from build123d import *

# Parameters (mm, degrees)
F2_SIZE2 = 1.1917535926
F2_SIZE  = 1
F3_SIZE2 = 1.1917535926
F3_SIZE  = 1
F4_SIZE  = 2
F5_SIZE2 = 1.1917535926
F5_SIZE  = 1
F6_SIZE2 = 1.1917535926
F6_SIZE  = 1


with BuildPart() as f1:
    # F0 (on Front) → F1 (revolve)
    with BuildSketch(Plane.XZ):
        Polygon((0, 30), (0, 6), (8, 6), (8, 16), (79.0824640741, 16), (91, 6), (99, 6), (99, 25), (94, 25), (92.8082464074, 24), (4, 24), (4, 30), align=None)
    revolve(axis=Axis((29.4127222821, 0, 0), (1, 0, 0)))

    # F2
    f2_edges = [f1.edges().sort_by_distance(p)[0] for p in [
        (0, 0, -6),
    ]]
    f2_side = f1.faces().sort_by_distance((0, 0, -29.151472))[0]
    chamfer(f2_edges, length=F2_SIZE, length2=F2_SIZE2, reference=f2_side)

    # F3
    f3_edges = [f1.edges().sort_by_distance(p)[0] for p in [
        (99, 0, -6),
    ]]
    f3_side = f1.faces().sort_by_distance((99, 0, -6.707107))[0]
    chamfer(f3_edges, length=F3_SIZE, length2=F3_SIZE2, reference=f3_side)

    # F4
    f4_edges = [f1.edges().sort_by_distance(p)[0] for p in [
        (99, 0, -25),
    ]]
    chamfer(f4_edges, length=F4_SIZE)

    # F5
    f5_edges = [f1.edges().sort_by_distance(p)[0] for p in [
        (0, 0, -30),
    ]]
    f5_side = f1.faces().sort_by_distance((0, 0, -7.848528))[0]
    chamfer(f5_edges, length=F5_SIZE, length2=F5_SIZE2, reference=f5_side)

    # F6
    f6_edges = [f1.edges().sort_by_distance(p)[0] for p in [
        (4, 0, -30),
    ]]
    f6_side = f1.faces().sort_by_distance((4, 0, -24.848528))[0]
    chamfer(f6_edges, length=F6_SIZE, length2=F6_SIZE2, reference=f6_side)


solid = f1.part
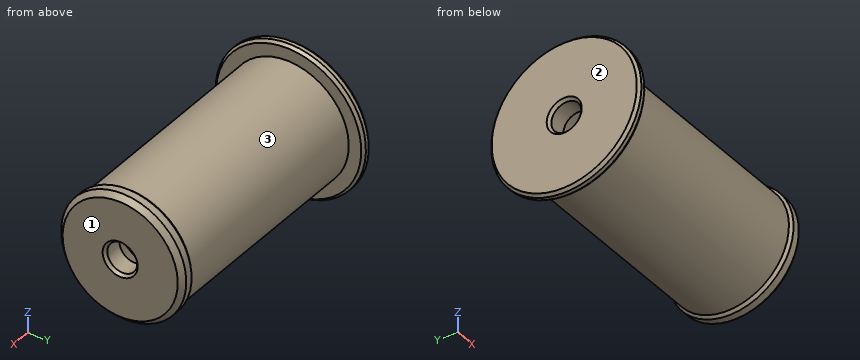
CAD build for the part. Positions are in the model's coordinates, mm. Face numbers are marked on the shaded views. Round coordinates to 2 decimals unless told otherwise and drop trailing zeros. Write each loop counter-clockwise with the first axis right and the second up, starting at its lowest first coordinate (ties: lowest second). Pieces come first, ordered by that corner, then holes. Notation, with made-up numbers: M 55,52.25 L 99,52.25 A20 cw 99,58.25 Z; hole C -34.75,57.5 d4. An arc over 180 degrees is marked long. Put each result on its own line as item: value. Start each with the question number.
1) Pull direction X, two halves, no side cores. Call the marked faces 1, 2 and 3: pulls with the +X half, pulls with the -X half, needs draft (parallel to the pull), parting line crosses it, or undercut.
2) Drill centre lines: probe 1 along Y at (x, z) = (5, 0); probe 2 along Z at (x, y) = (94, 0); probe 3 along Z at (x, y) = (62, 0). Where is each one in solid material? Low to high. Write a range as [from, to].
3) Saw through at C-C, the plane x = 36. Write the cut outline in (y, z), and give its area (3 significant figures).
4) Pin check, flat tips, straight feed: pin 1 Ø7 at (y, z) = (0, 0) entering from -X; pin 2 Ø12 at (x, y) = (17, -22) entering from +Z; pin 3 Ø1.5 at (y, z) = (-12.5, 18.5) entering from -X; pin 4 Ø10 at (x, z) = (77.5, -2) entering from -Y. Stop position of each tip, or through.
Resolved:
1. face 1: pulls with the +X half
1. face 2: pulls with the -X half
1. face 3: undercut
2. probe 1: [-24, -6], [6, 24]
2. probe 2: [-25, -6], [6, 25]
2. probe 3: [-24, -16], [16, 24]
3. outline: C 0,0 d48; hole C 0,0 d32
3. area: 1,010 mm²
4. pin 1: through
4. pin 2: z = 17.89
4. pin 3: x = 0
4. pin 4: y = -24
